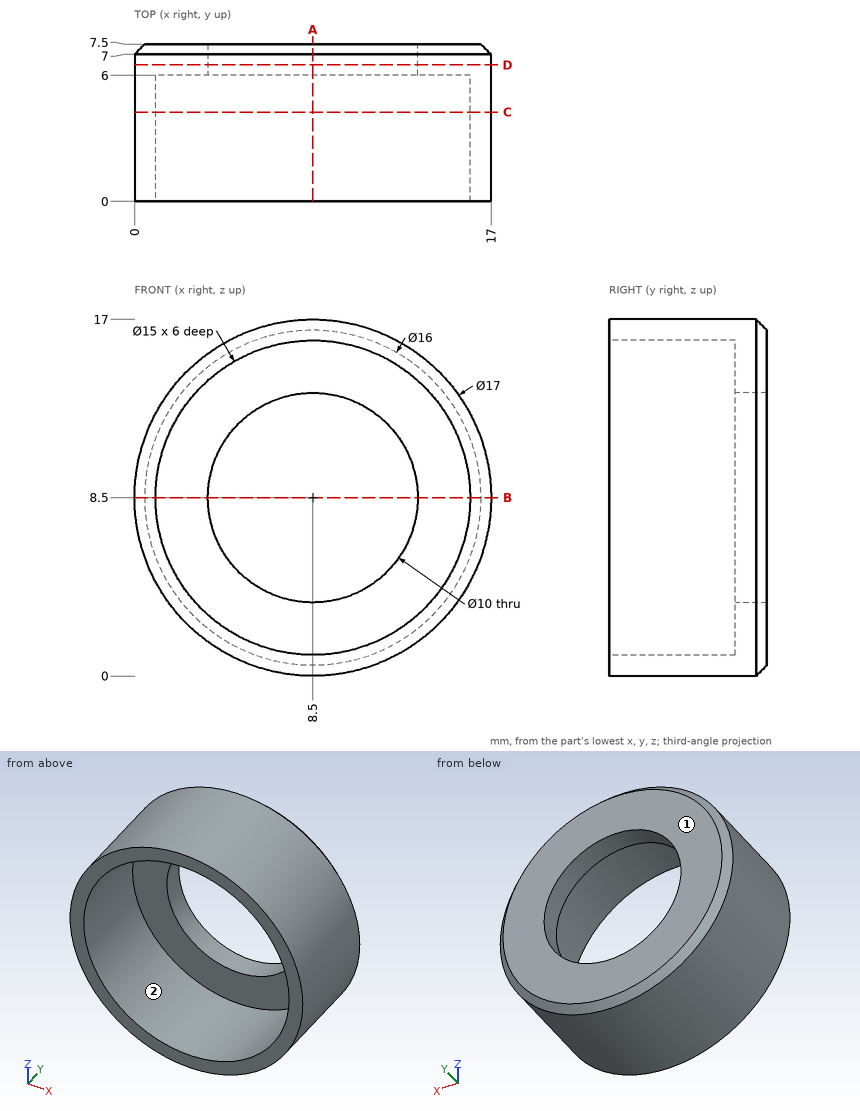
Design review of the part shown in the three views and the two pictorial views. Dimensions are in mm from the part's minimum x, y and z. A direction names the side the tool comes from. Round coordinates to 2 decimals unless told otherwise and drop trailing zeros. Loops run counter-clockwise (first coordinate to the right, second up) from the corner with the lowest first, then second, coordinate; pieces in that order, holes last. Notation, with made-up numbers: M 19.25,-36.5 L 78.25,-36.5 A32 cw 78.25,-4.5 Z; hole C 15,-9.5 d5. An arc over 180 degrees is marked long. Put each result on its own line as item: value.
Q1. To check wall thickness, follow L1, parallel to Z at x = 8.5, y = 6.9; L2, parallel to Z at x = 8.5, y = 2.5. State the ranges of each line that lie inside material, in increasing order.
Result set:
L1: z = 0 to 3.5, 13.5 to 17
L2: z = 0 to 1, 16 to 17
Q2. For pin 1 (4 mm diameter, centred on x = 3, y = 3, fed in from +Z); pin 2 (3 mm diameter, centred on y = 5.5, z = 5, fed in from -X); pin 3 (4.5 mm diameter, centred on x = 5.5, z = 11.5, fed in from -Y), all flat-tipped, find the tip position at first contact; note any pin that passes through.
Result set:
pin 1: stops at z = 16.25
pin 2: stops at x = 0.24
pin 3: stops at y = 6
Q3. Consider section C-C, the plane y = 4.25. Give the boundary of the cut face in (x, z), then the cut area to 3 significant figures.
Result set:
outline: C 8.5,8.5 d17; hole C 8.5,8.5 d15
area: 50.3 mm²
Q4. Consider section B-B, the plane z = 8.5. Give the boundary of the cut face in (x, y), then the cut area to 4 significant figures.
Result set:
outline: M 0,0 L 1,0 L 1,6 L 3.5,6 L 3.5,7.5 L 0.5,7.5 L 0,7 Z; M 13.5,6 L 16,6 L 16,0 L 17,0 L 17,7 L 16.5,7.5 L 13.5,7.5 Z
area: 22.25 mm²
Q5. Consider section A-A, the plane x = 8.5. Give the boundary of the cut face in (y, z).
Result set:
outline: M 0,0 L 7,0 L 7.5,0.5 L 7.5,3.5 L 6,3.5 L 6,1 L 0,1 Z; M 0,16 L 6,16 L 6,13.5 L 7.5,13.5 L 7.5,16.5 L 7,17 L 0,17 Z
Q6. Consider section D-D, the plane y = 6.5. Give the boundary of the cut face in (x, z).
Result set:
outline: C 8.5,8.5 d17; hole C 8.5,8.5 d10
Q7. Machinability: for the marked faces 1 and 2, which of the approach directions +Z, -Z, +X, -X, +Y, -Y give a long, thin tool a straight path to every point of the face, cutting with its end or side? Answer none if there is none.
Result set:
face 1: +Z, -Z, +X, -X, +Y
face 2: -Y
